from build123d import *

# Parameters (mm, degrees)
SKETCH1_R           = 1.65
BOSS_EXTRUDE1_DEPTH = 10.6
SKETCH2_OUTSIDE_W   = 66.756
SKETCH2_OUTSIDE_H   = 66.356
SKETCH2_OUTSIDE_W_2 = 50.4
SKETCH2_OUTSIDE_H_2 = 29.8
CUT_EXTRUDE1_DEPTH  = 4.6
CUT_EXTRUDE2_DEPTH  = 8.4
SKETCH4_OUTSIDE_W   = 66.756
SKETCH4_OUTSIDE_H   = 26.956
CUT_EXTRUDE3_DEPTH  = 50


with BuildPart() as part:
    # Sketch1 → Boss-Extrude1 (new body)
    with BuildSketch(Plane.XY):
        with BuildLine():
            Line((-17.536336397, 19.751180304), (-17.536336397, 23))
            ThreePointArc((-17.536336397, 23), (-16.950549959, 24.414213562), (-15.536336397, 25))
            Line((-15.536336397, 25), (23.2, 25))
            ThreePointArc((23.2, 25), (24.614213562, 24.414213562), (25.2, 23))
            Line((25.2, 23), (25.2, -23))
            ThreePointArc((25.2, -23), (24.614213562, -24.414213562), (23.2, -25))
            Line((23.2, -25), (-23.2, -25))
            ThreePointArc((-23.2, -25), (-24.614213562, -24.414213562), (-25.2, -23))
            Line((-25.2, -23), (-25.2, 14.9))
            ThreePointArc((-25.2, 14.9), (-25.01741556, 15.476048437), (-24.536336397, 15.841741912))
            Line((-24.536336397, 15.841741912), (-18.863663603, 17.867696481))
            ThreePointArc((-18.863663603, 17.867696481), (-17.901505276, 18.599083431), (-17.536336397, 19.751180304))
        make_face()
        with Locations((0, 20)):
            Circle(SKETCH1_R, mode=Mode.SUBTRACT)
        with Locations((0, -20)):
            Circle(SKETCH1_R, mode=Mode.SUBTRACT)
        with BuildLine():
            Line((-19.15, -13.7), (-19.15, 13.7))
            ThreePointArc((-19.15, 13.7), (-18.798528137, 14.548528137), (-17.95, 14.9))
            Line((-17.95, 14.9), (17.95, 14.9))
            ThreePointArc((17.95, 14.9), (18.798528137, 14.548528137), (19.15, 13.7))
            Line((19.15, 13.7), (19.15, -13.7))
            ThreePointArc((19.15, -13.7), (18.798528137, -14.548528137), (17.95, -14.9))
            Line((17.95, -14.9), (-17.95, -14.9))
            ThreePointArc((-17.95, -14.9), (-18.798528137, -14.548528137), (-19.15, -13.7))
        make_face(mode=Mode.SUBTRACT)
    extrude(amount=BOSS_EXTRUDE1_DEPTH)

    # Sketch2 outside → Cut-Extrude1 (cut)
    with BuildSketch(Plane.XY.offset(10.6)):
        Rectangle(SKETCH2_OUTSIDE_W, SKETCH2_OUTSIDE_H)
        Rectangle(SKETCH2_OUTSIDE_W_2, SKETCH2_OUTSIDE_H_2, mode=Mode.SUBTRACT)
    extrude(amount=-CUT_EXTRUDE1_DEPTH, mode=Mode.SUBTRACT)

    # Sketch3 → Cut-Extrude2 (cut)
    with BuildSketch(Plane.XY.offset(10.6)):
        with BuildLine():
            Line((-20.8, -14.75), (-20.8, 14.75))
            ThreePointArc((-20.8, 14.75), (-20.448528137, 15.598528137), (-19.6, 15.95))
            Line((-19.6, 15.95), (19.6, 15.95))
            ThreePointArc((19.6, 15.95), (20.448528137, 15.598528137), (20.8, 14.75))
            Line((20.8, 14.75), (20.8, -14.75))
            ThreePointArc((20.8, -14.75), (20.448528137, -15.598528137), (19.6, -15.95))
            Line((19.6, -15.95), (-19.6, -15.95))
            ThreePointArc((-19.6, -15.95), (-20.448528137, -15.598528137), (-20.8, -14.75))
        make_face()
    extrude(amount=-CUT_EXTRUDE2_DEPTH, mode=Mode.SUBTRACT)

    # Sketch4 outside → Cut-Extrude3 (cut)
    with BuildSketch(Plane.XZ.offset(25)):
        with Locations((0, 5.3)):
            Rectangle(SKETCH4_OUTSIDE_W, SKETCH4_OUTSIDE_H)
        Polygon((-24.1, 7.4), (-24.65, 7.95), (-24.1, 10.6), (-21.79058809, 10.6), (-20.79058809, 6), (20.79058809, 6), (21.79058809, 10.6), (24.1, 10.6), (24.65, 7.95), (24.1, 7.4), (24.1, 6), (25.2, 6), (25.2, 0), (-25.2, 0), (-25.2, 6), (-24.1, 6), align=None, mode=Mode.SUBTRACT)
    extrude(amount=-CUT_EXTRUDE3_DEPTH, mode=Mode.SUBTRACT)


solid = part.part
Model file for the job. Use its own axes, mm. A direction names the side the tool comes from. Give positions to 0.01 mm unless a question says otherwise; leave off trailing zeros. Order: outer loops, then holes, each group sorted by start corner. A loop starts at its lowest first (then second) coordinate and runs counter-clockwise, first axis right, second up. Notation, with made-up numbers: (44.25, 10.5) - (71.25, 10.5) arc R13 cw to (71.25, 25.5) - close; hole circle Ø6 at (14.5, 9). An arc over 180 degrees is marked (long way). Return JSON: item names as keys, results as strings.
1) Cut at C-C, the plane z = 5. Give the cut face in (x, y).
Geometry says:
{"outline": "(-25.2, -23) arc R2 ccw to (-23.2, -25) - (23.2, -25) arc R2 ccw to (25.2, -23) - (25.2, 23) arc R2 ccw to (23.2, 25) - (-15.54, 25) arc R2 ccw to (-17.54, 23) - (-17.54, 19.75) arc R2 cw to (-18.86, 17.87) - (-24.54, 15.84) arc R1 ccw to (-25.2, 14.9) - close; hole (-20.8, -14.75) arc R1.2 ccw to (-19.6, -15.95) - (19.6, -15.95) arc R1.2 ccw to (20.8, -14.75) - (20.8, 14.75) arc R1.2 ccw to (19.6, 15.95) - (-19.6, 15.95) arc R1.2 ccw to (-20.8, 14.75) - close; hole circle Ø3.3 at (0, -20); hole circle Ø3.3 at (0, 20)"}
2) Pull direction X, two halves, no side cores. Call faces 6 (the cylindrical face through (-16.966, 24.399, 2.958)), 7 (the flat face through (19.15, 0, 1)), 8 (the flat face through (-23, 14.9, 8)): pulls with the +X half, pulls with the -X half, needs draft (parallel to the pull), parting line crosses it, or undercut.
Geometry says:
{"face 6": "pulls with the -X half", "face 7": "undercut", "face 8": "needs draft"}
3) Cut at A-A, the plane y = -8.5. Give the cut face in (x, z).
Geometry says:
{"outline": "(-25.2, 0) - (-19.15, 0) - (-19.15, 2.2) - (-20.8, 2.2) - (-20.8, 6.04) - (-21.79, 10.6) - (-24.1, 10.6) - (-24.65, 7.95) - (-24.1, 7.4) - (-24.1, 6) - (-25.2, 6) - close; (19.15, 0) - (25.2, 0) - (25.2, 6) - (24.1, 6) - (24.1, 7.4) - (24.65, 7.95) - (24.1, 10.6) - (21.79, 10.6) - (20.8, 6.04) - (20.8, 2.2) - (19.15, 2.2) - close"}
4) 3-axis set-ups, long thin cutter, end or side, ignore diameter. For faces 1 (the flat face through (23, -14.9, 8)), 2 (the flat face through (-24.1, 0, 7)), 3 (the flat face through (23, 14.9, 8)), 4 (the flat face through (-20.8, 0, 4)), 5 (the flat face through (21.284, -0.209, 8.268)): which of +Z, -Z, +X, -X, +Y, -Y reach the whole face in a straight line?
Geometry says:
{"face 1": "+Z, +X, -X, -Y", "face 2": "-X, +Y, -Y", "face 3": "+Z, +X, -X, +Y", "face 4": "+Z", "face 5": "+Z, +Y, -Y"}
5) Flat gauge pins, fed straight in: P1, Ø1.1, axis at y = 7, z = 7, coming from the +X side; P2, Ø8, axis at x = -20, y = -9.5, coming from the +Z side; P3, Ø16, axis at x = 4, y = 7, coming from the +Z side; P4, Ø3, axis at y = -11, z = 9.5, coming from the +X side. Where does each tip first touch, or does it go through?
Geometry says:
{"P1": "x = 24.25", "P2": "z = 10.6", "P3": "z = 2.2", "P4": "x = 24.64"}
6) Cut at D-D, the plane x = 0. Give the cut face in (y, z), plus the area to 3 significant figures.
Geometry says:
{"outline": "(-25, 0) - (-21.65, 0) - (-21.65, 6) - (-25, 6) - close; (-18.35, 0) - (-14.9, 0) - (-14.9, 2.2) - (-15.95, 2.2) - (-15.95, 6) - (-18.35, 6) - close; (14.9, 0) - (18.35, 0) - (18.35, 6) - (15.95, 6) - (15.95, 2.2) - (14.9, 2.2) - close; (21.65, 0) - (25, 0) - (25, 6) - (21.65, 6) - close", "area": "73.6 mm²"}
7) Cut at B-B, the plane x = -8. Give the cut face in (y, z).
Geometry says:
{"outline": "(-25, 0) - (-14.9, 0) - (-14.9, 2.2) - (-15.95, 2.2) - (-15.95, 6) - (-25, 6) - close; (14.9, 0) - (25, 0) - (25, 6) - (15.95, 6) - (15.95, 2.2) - (14.9, 2.2) - close"}
8) Probe line 1 (Y direction, x = 0, z = 4.85); line 2 (X direction, y = -20, z = 3.6); line 3 (X direction, y = 5.5, z = 0.75). List the from-to ranges inside material, lowest first. Write a range as from..to.
Geometry says:
{"line 1": "-25..-21.65, -18.35..-15.95, 15.95..18.35, 21.65..25", "line 2": "-25.2..-1.65, 1.65..25.2", "line 3": "-25.2..-19.15, 19.15..25.2"}
